Could you check a few things on this model? Use its own coordinates, in mm. A direction names the side the tool comes from. Coordinates: 2 decimals unless noted, no trailing zeros. Order: outer loops, then holes, each group sorted by start corner. A loop starts at its lowest first (then second) coordinate and runs counter-clockwise, first axis right, second up. Notation, with made-up numbers: (87.25, 28.5) - (141.25, 28.5) arc R22 cw to (141.25, 56.5) - close; hole circle Ø11 at (-34.75, 47). An arc over 180 degrees is marked (long way). Answer as CSV lines item,"result". Start each with the question number.
1. I want a section at D-D, the plane z = 30. List the corners of the cut face in (x, y) for me.
2. I want a section at C-C, the plane y = -11. List the corners of the cut face in (x, z) for me, and give its area (3 significant figures).
3. I want a section at B-B, the plane x = 22. List the corners of the cut face in (y, z) for me.
4. I need wall thicknesses on probe 1 along Z at (x, y) = (22, 12.5); probe 2 along X at (y, z) = (-2.5, 32.5); probe 3 along Y at (x, z) = (-3, 27). Which ranges of each line are inside material? Lowest first, please.
5. I want a section at A-A, the plane z = 23.5. List the corners of the cut face in (x, y) for me, and give its area (3 significant figures).
6. For faces 5 (the face through (-16.801, 23, 2)), 6 (the face through (-23, -16.8, 2)), 7 (the face through (16.799, 23, 2)), 8 (the face through (-5.5, 13.6, 20.2)), which set-ups out of +Z, -Z, +X, -X, +Y, -Y let a thin tool reach every point of the face, with its end or its side?
7. Thinking about a two-plate mould opening in X: for faces 1 (the face through (10, 11, 5)), 2 (the face through (17.93, -7.36, 31.38)), 3 (the face through (16.799, -23, 2)), 4 (the face through (-6.56, 17.12, 31.38)), which applies, released by +X, released by -X, zero draft, split by the parting line, or undercut?
8. For pin 1 (4 mm diameter, centred on x = -19, z = 16, fed in from -Y); pin 2 (1.8 mm diameter, centred on y = -23, z = 2, fed in from -X); pin 3 (4 mm diameter, centred on y = -23.5, z = 2.5, fed in from +X); pin 4 (4 mm diameter, centred on x = -9.5, z = 23, fed in from -Y), each with a flat end and sliding along its axis, tell me the tip position at first contact or that it passes through.
Autodesk Inventor part; units mm, degrees
ref_plane "YZ Plane" through (0, 0, 0) normal (1, 0, 0) x (0, 1, 0)
ref_plane "XZ Plane" through (0, 0, 0) normal (0, 1, 0) x (-1, 0, 0)
ref_plane "XY Plane" through (0, 0, 0) normal (0, 0, 1) x (1, 0, 0)
sketch "草图1" plane through (0, 0, 0) normal (0, 0, 1) x (1, 0, 0)
  line L0 (24.9, 0) -> (24.9, 16.8)
  line L1 (24.9, 0) -> (41.7, 0) construction
  line L2 (24.9, 16.8) -> (21.24, 16.8)
  line L3 (21.24, 16.8) -> (16.7994, 21.2406)
  line L4 (16.7994, 21.2406) -> (16.7994, 24.9006)
  line L5 (16.7994, 24.9006) -> (-0.0006, 24.9006)
  line L6 (24.9, 0) -> (24.9, -16.8)
  line L7 (24.9, -16.8) -> (21.24, -16.8)
  line L8 (21.24, -16.8) -> (16.7994, -21.2406)
  line L9 (16.7994, -21.2406) -> (16.7994, -24.9006)
  line L10 (16.7994, -24.9006) -> (-0.0006, -24.9006)
  line L11 (-0.0006, -24.9006) -> (-16.8006, -24.9006)
  line L12 (-16.8006, -24.9006) -> (-16.8006, -21.2406)
  line L13 (-16.8006, -21.2406) -> (-21.2413, -16.8)
  line L14 (-21.2413, -16.8) -> (-24.9013, -16.8)
  line L15 (-24.9013, -16.8) -> (-24.9013, 0)
  line L16 (-24.9013, 0) -> (-24.9013, 16.8)
  line L17 (-24.9013, 16.8) -> (-21.2413, 16.8)
  line L18 (-21.2413, 16.8) -> (-16.8006, 21.2406)
  line L19 (-16.8006, 21.2406) -> (-16.8006, 24.9006)
  line L20 (-16.8006, 24.9006) -> (-0.0006, 24.9006)
  point P0 (0, 0)
extrude "拉伸1" add sketch "草图1" along normal blind 5
sketch "草图2" plane through (0, 0, 5) normal (0, 0, 1) x (1, 0, 0)
  point P0 (0, 0)
sketch "草图3" plane through (0, 0, 5) normal (0, 0, 1) x (1, 0, 0)
  line L0 (21.24, -16.8) -> (-16.8006, 21.2406)
  line L1 (-16.8006, 24.9006) -> (-16.8006, 21.2406)
  line L2 (-16.8006, 24.9006) -> (-11.8006, 24.9006)
  line L3 (16.7994, 24.9006) -> (-16.8006, 24.9006)
  line L4 (21.24, -16.8) -> (24.9, -16.8)
  line L5 (24.9, -16.8) -> (24.9, -11.8)
  line L6 (24.9, -16.8) -> (24.9, 16.8)
  line L7 (24.9, -11.8) -> (-11.8006, 24.9006)
  point P0 (0, 0)
extrude "拉伸2" add sketch "草图3" along normal blind 30
sketch "草图4" plane through (-11.8006, 24.9006, 5) normal (0.7071, 0.7071, 0) x (-0.7071, 0.7071, 0)
  line L0 (-51.9025, 0) -> (-51.9025, 30)
  line L1 (0, 0) -> (0, 30)
  line L2 (-51.9025, 30) -> (0, 0) construction
  line L3 (-51.9025, 30) -> (0, 30)
  line L4 (0, 30) -> (-51.9025, 0) construction
  point P0 (-25.9517, -5)
  point P1 (-25.9513, 15)
hole "孔1" at (6.5497, 6.5503, 20) direction (-0.7071, -0.7071, 0) diameter 24.5 end through all
sketch "草图5" plane through (-11.8006, 24.9006, 5) normal (0.7071, 0.7071, 0) x (-0.7071, 0.7071, 0)
  line L0 (-51.9025, 0) -> (-51.9025, 30)
  line L1 (0, 0) -> (-51.9025, 0)
  line L2 (0, 0) -> (0, 30)
  point P0 (-25.9517, -5)
  point P1 (-25.9513, 15)
  point P2 (-12.9646, 7.4936)
hole "孔2" at (6.5497, 6.5503, 20) direction (-0.7071, -0.7071, 0) diameter 0.01 end through all
sketch "草图6" plane through (0, 0, 35) normal (0, 0, 1) x (1, 0, 0)
  line L0 (-11.8006, 24.9006) -> (-16.8006, 24.9006)
  line L1 (-16.8006, 24.9006) -> (-16.8006, 21.2406)
  line L2 (-16.8006, 24.9006) -> (-16.8006, 21.2406)
  line L3 (21.24, -16.8) -> (-16.8006, 21.2406)
  line L4 (-16.8006, 21.2406) -> (21.24, -16.8)
  line L5 (24.9, -16.8) -> (24.9, 16.8)
  line L6 (-16.8006, 24.9006) -> (24.9, -16.8)
  line L7 (24.9, -16.8) -> (21.24, -16.8)
  point P0 (0, 0)
extrude "拉伸3" cut sketch "草图6" against normal blind 30
sketch "草图7" plane through (-11.8006, 24.9006, 5) normal (0.7071, 0.7071, 0) x (-0.7071, 0.7071, 0)
  line L0 (-51.9025, 0) -> (-51.9025, 30)
  line L1 (0, 0) -> (0, 30)
  line L2 (-51.9025, 30) -> (0, 0)
  line L3 (-51.9025, 0) -> (0, 30)
  line L4 (-25.9513, 15) -> (-43.2669, 25.0085)
  line L5 (-25.9513, 15) -> (-7.1239, 25.8823)
  line L6 (-25.9513, 15) -> (-8.6357, 25.0085)
  line L7 (-25.9513, 15) -> (-41.7093, 5.8917)
  line L8 (-25.9513, 15) -> (-43.2669, 4.9915)
  point P0 (-25.9517, -5)
hole "孔3" at (18.7937, -5.6937, 30.0085) at (-5.6943, 18.7943, 30.0085) direction (-0.7071, -0.7071, 0) diameter 2.97 end through all
sketch "草图8" plane through (-11.8006, 24.9006, 5) normal (0.7071, 0.7071, 0) x (-0.7071, 0.7071, 0)
  circle A0 centre (-43.2669, 4.9915) radius 1.485
  line L0 (-43.2669, 4.9915) -> (-43.2669, 6.9915)
  point P0 (-25.9517, -5)
  dimension "d43" = 2
hole "孔4" at (18.7937, -5.6937, 11.9915) direction (-0.7071, -0.7071, 0) diameter 2.97 end through all
equation "\"d41\" = Thickness"
equation "\"d49\" = Thickness"
equation "\"BendRadius\" = Thickness"
equation "\"BendReliefWidth\" = Thickness"
equation "\"BendReliefDepth\" = 0.5 * Thickness"
equation "\"CornerReliefSize\" = 4 * Thickness"
equation "\"MinimumRemnant\" = 2 * Thickness"
equation "\"TransitionRadius\" = BendRadius"
equation "\"JacobiRadiusSize\" = BendRadius"
equation "\"GapSize\" = Thickness"
properties part number "可调底座"
Solved:
1,outline,"(-16.8, 24.9) - (-9.24, 17.34) - (-6.74, 19.84) - (-11.8, 24.9) - close; (-7.14, 15.24) - (-0.95, 9.05) - (1.55, 11.55) - (-4.64, 17.74) - close; (9.05, -0.95) - (15.24, -7.14) - (17.74, -4.64) - (11.55, 1.55) - close; (17.34, -9.24) - (24.9, -16.8) - (24.9, -11.8) - (19.84, -6.74) - close"
2,outline,"(-24.9, 0) - (24.9, 0) - (24.9, 5) - (24.1, 5) - (24.1, 35) - (19.1, 35) - (19.1, 5) - (-24.9, 5) - close"
2,area,"399 mm2"
3,outline,"(-16.8, 0) - (16.8, 0) - (16.8, 5) - (-8.9, 5) - (-8.9, 35) - (-13.9, 35) - (-13.9, 5) - (-16.8, 5) - close"
4,probe 1,"z = 0 to 5"
4,probe 2,"x = 10.6 to 15.6"
4,probe 3,"y = 11.22 to 16.1"
5,outline,"(-16.8, 24.9) - (-4.25, 12.35) - (-1.75, 14.85) - (-11.8, 24.9) - close; (12.35, -4.25) - (24.9, -16.8) - (24.9, -11.8) - (14.85, -1.75) - close"
5,area,"113 mm2"
6,face 5,"+Z, -Z, -X, +Y"
6,face 6,"+Z, -Z, -X, -Y"
6,face 7,"+Z, -Z, +X, +Y"
6,face 8,"+Z, -X, -Y"
7,face 1,"zero draft"
7,face 2,"undercut"
7,face 3,"released by +X"
7,face 4,"undercut"
8,pin 1,"passes through"
8,pin 2,"stops at x = -16.8"
8,pin 3,"stops at x = 16.8"
8,pin 4,"stops at y = 15.6"
